The figure shows three views and two pictorial views of one solid part (mm, origin at its lowest corner). Answer the questions. Coordinates: 2 decimals unless noted, no trailing zeros. Loops run counter-clockwise (first coordinate to the right, second up) from the corner with the lowest first, then second, coordinate; pieces in that order, holes last. Notation, with made-up numbers: (52, 44) - (75, 44) arc R20 cw to (75, 61) - close; hole circle Ø7 at (39, -19.75). An arc over 180 degrees is marked (long way). Write each question's results on one line, items separated by ' | '. Start each with the question number.
Item 1: Each of these flat-tipped pins is pushed along its axis until it touches: pin 1 Ø10 at (x, z) = (85, 29) entering from -Y (1 decimal); pin 2 Ø1.5 at (x, z) = (42, 22) entering from -Y; pin 3 Ø3 at (y, z) = (43, 66) entering from -X; pin 4 Ø2 at (x, y) = (35.5, 34) entering from -Z. Where does it stop, or does it pass through?
Item 2: Consider probe 1 along X at (y, z) = (47.5, 31) (1 decimal); probe 2 along Y at (x, z) = (48, 54.5); probe 3 along Y at (x, z) = (53, 24.5) (1 decimal). Determine where each line is inside the solid, lowest interval first. Write a range as [from, to].
Item 3: Section A-A, the plane z = 70 is taken. Write down the section's boundary in (x, y).
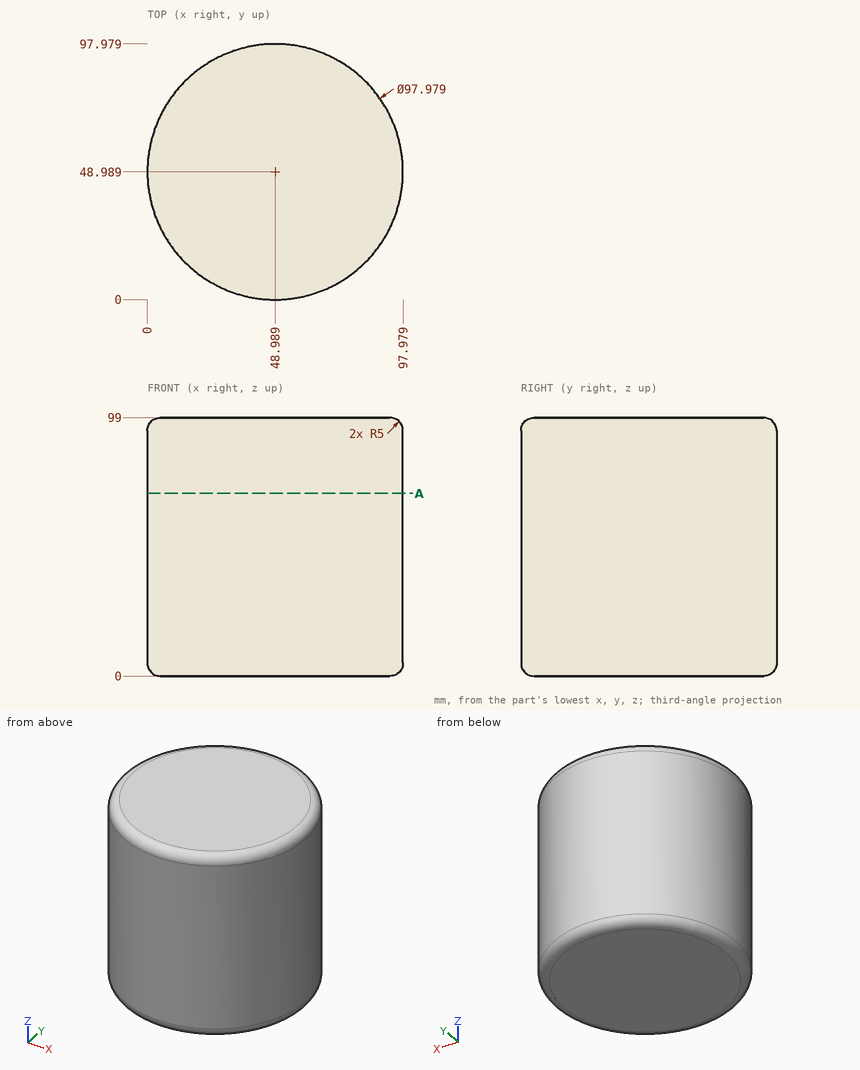
Answer key:
1) pin 1: stops at y = 11.1 | pin 2: stops at y = 0.4 | pin 3: stops at x = 0.21 | pin 4: stops at z = 0
2) probe 1: x = [0, 98] | probe 2: y = [0.01, 97.97] | probe 3: y = [0.2, 97.8]
3) outline: circle Ø97.98 at (48.99, 48.99)
